Design review of the part built by this model. Coordinates are the model's own, in mm. Face numbers are marked on the shaded views. A direction names the side the tool comes from. Coordinates: 2 decimals unless noted, no trailing zeros. Loops run counter-clockwise (first coordinate to the right, second up) from the corner with the lowest first, then second, coordinate; pieces in that order, holes last. Notation, with made-up numbers: (5.25, 69.25) -> (34.25, 69.25) arc R32 ccw to (34.25, 99.25) -> close; hole circle Ø5 at (-6, 56.5). An arc over 180 degrees is marked (long way). Answer as a JSON object with one key per item and string values.
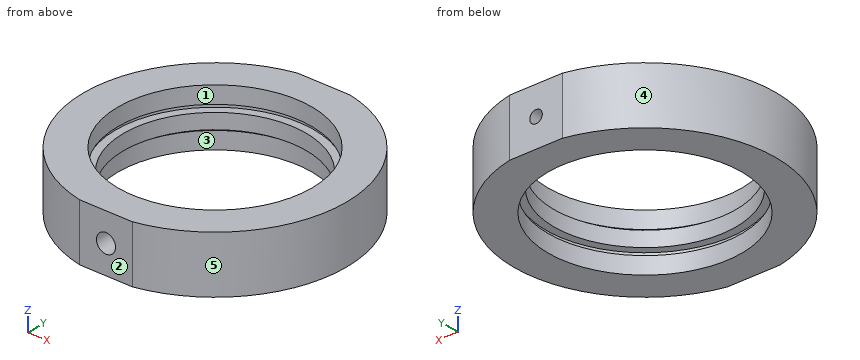
```python
from build123d import *

# Parameters (mm, degrees)
SKETCH_2_W             = 64.02174429
SKETCH_2_H             = 9.248919907
CUT_EXTRUDE_1_DEPTH    = 49
HOLE_WIZARD_M4_2_D     = 3.3
HOLE_WIZARD_M4_2_DEPTH = 5.5
HOLE_WIZARD_M4_2_TIP   = 0.991420021
HOLE_WIZARD_M6_2_D     = 5
HOLE_WIZARD_M6_2_DEPTH = 5.5
HOLE_WIZARD_M6_2_TIP   = 1.502151548


with BuildPart() as part:
    # 草图1 → 旋转1 (revolve)
    with BuildSketch(Plane(origin=(0, 0, 0), x_dir=(1, 0, 0), z_dir=(0, 1, 0)), mode=Mode.PRIVATE) as revolve_1_sk:
        Polygon((34.5, 7.5), (34.5, -7.5), (25.5, -7.5), (25.5, -3), (26.1, -3), (26.1, -2), (25.5, -2), (24, -2), (24, 2), (25.5, 2), (26.1, 2), (26.1, 3), (25.5, 3), (25.5, 7.5), align=None)
    revolve(revolve_1_sk.sketch.rotate(Axis((0, 0, -31.9390681), (0, 0, 1)), 180), axis=Axis((0, 0, -31.9390681), (0, 0, 1)))  # turned: the seam where the file's is

    # 草图2 → 切除-拉伸1 (cut)
    with BuildSketch(Plane.XY.offset(7.5)):
        with Locations((-1.141100508, 38.424459954)):
            Rectangle(SKETCH_2_W, SKETCH_2_H)
        with Locations((-1.141100508, -38.424459954)):
            Rectangle(SKETCH_2_W, SKETCH_2_H)
    extrude(amount=-CUT_EXTRUDE_1_DEPTH, mode=Mode.SUBTRACT)

    # M4 螺纹孔2
    with Locations(Plane(origin=(0, 33.8, 0), x_dir=(1, 0, 0), z_dir=(0, 1, 0))):
        with Locations((0, 0)):
            Hole(HOLE_WIZARD_M4_2_D / 2, depth=HOLE_WIZARD_M4_2_DEPTH)
            with Locations((0, 0, -(HOLE_WIZARD_M4_2_DEPTH + HOLE_WIZARD_M4_2_TIP / 2))):  # 118° drill point
                Cone(0, HOLE_WIZARD_M4_2_D / 2, HOLE_WIZARD_M4_2_TIP, mode=Mode.SUBTRACT)

    # M6 螺纹孔2
    with Locations(Plane(origin=(0, -33.8, 0), x_dir=(-1, 0, 0), z_dir=(0, -1, 0))):
        with Locations((0, 0)):
            Hole(HOLE_WIZARD_M6_2_D / 2, depth=HOLE_WIZARD_M6_2_DEPTH)
            with Locations((0, 0, -(HOLE_WIZARD_M6_2_DEPTH + HOLE_WIZARD_M6_2_TIP / 2))):  # 118° drill point
                Cone(0, HOLE_WIZARD_M6_2_D / 2, HOLE_WIZARD_M6_2_TIP, mode=Mode.SUBTRACT)


solid = part.part
```
1) Add section B-B, the plane z = 6. Give the boundary of the cut face in (x, y), and give its area (3 significant figures).
Completed:
{"outline": "(-6.91, -33.8) -> (6.91, -33.8) arc R34.5 ccw to (6.91, 33.8) -> (-6.91, 33.8) arc R34.5 ccw to start; hole circle Ø51 at (0, 0)", "area": "1,680 mm²"}
2) Add section C-C, the plane x = 15. Give the boundary of the cut face in (y, z) (3 decimals).
Completed:
{"outline": "(-31.068, -7.5) -> (-20.622, -7.5) -> (-20.622, -3) -> (-21.359, -3) -> (-21.359, -2) -> (-18.735, -2) -> (-18.735, 2) -> (-21.359, 2) -> (-21.359, 3) -> (-20.622, 3) -> (-20.622, 7.5) -> (-31.068, 7.5) -> close; (18.735, -2) -> (21.359, -2) -> (21.359, -3) -> (20.622, -3) -> (20.622, -7.5) -> (31.068, -7.5) -> (31.068, 7.5) -> (20.622, 7.5) -> (20.622, 3) -> (21.359, 3) -> (21.359, 2) -> (18.735, 2) -> close"}
3) Clearance check with flat-ended pins moving along their axes: pin 1 Ø1 at (y, z) = (14, -2) entering from +X; pin 2 Ø6 at (y, z) = (-18, -4.5) entering from +X; pin 3 Ø3 at (x, z) = (0, 0) entering from -Y. State where each tip first meets the part, or that it passes through.
Completed:
{"pin 1": "x = 31.75", "pin 2": "x = 31.07", "pin 3": "y = -27.7"}
4) The part is to be moulded in two halves that separate along X. For the marked faces 3, 4 and 5, say which applies: pulls with the +X half, pulls with the -X half, needs draft (parallel to the pull), parting line crosses it, or undercut.
Completed:
{"face 3": "undercut", "face 4": "pulls with the -X half", "face 5": "pulls with the +X half"}
5) Add section A-A, the plane y = 0. Give the boundary of the cut face in (x, z), and give its area (3 significant figures).
Completed:
{"outline": "(-34.5, -7.5) -> (-25.5, -7.5) -> (-25.5, -3) -> (-26.1, -3) -> (-26.1, -2) -> (-24, -2) -> (-24, 2) -> (-26.1, 2) -> (-26.1, 3) -> (-25.5, 3) -> (-25.5, 7.5) -> (-34.5, 7.5) -> close; (24, -2) -> (26.1, -2) -> (26.1, -3) -> (25.5, -3) -> (25.5, -7.5) -> (34.5, -7.5) -> (34.5, 7.5) -> (25.5, 7.5) -> (25.5, 3) -> (26.1, 3) -> (26.1, 2) -> (24, 2) -> close", "area": "280 mm²"}
6) Wall thickness on probe 1 along Y at (x, z) = (0, -2.65); probe 2 along Y at (x, z) = (0, 5.25); probe 3 along X at (y, z) = (-10.5, -4.75): over which ranges is each line inside the solid? List them lowest first.
Completed:
{"probe 1": "-33.8 to -26.1, 26.1 to 33.8", "probe 2": "-33.8 to -25.5, 25.5 to 33.8", "probe 3": "-32.86 to -23.24, 23.24 to 32.86"}
7) For the marked faces 1 and 2, list the 3-axis set-ups (+Z, -Z, +X, -X, +Y, -Y) from which the entire face can be reached by the end or side of a thin tool; tool diameter is ignored.
Completed:
{"face 1": "+Z", "face 2": "+Z, -Z, +X, -X, -Y"}
8) Add section D-D, the plane x = 30.5. Give the boundary of the cut face in (y, z), and give its area (3 significant figures).
Completed:
{"outline": "(-16.12, -7.5) -> (16.12, -7.5) -> (16.12, 7.5) -> (-16.12, 7.5) -> close", "area": "484 mm²"}
